from build123d import *

# Parameters (mm, degrees)
F0_W     = 38
F0_H     = 10
F1_DEPTH = 5
F2_R     = 1.5
F3_DEPTH = 5
F4_W     = 8
F4_H     = 5
F5_DEPTH = 5
F6_R     = 1.5
F7_DEPTH = 5
F8_R     = 4.99999


# Not quite as in the source:
# - a fillet or chamfer is up to 0.001 mm smaller than in the source, because OpenCascade refuses the exact size
# - a feature names something its author has since deleted; it is built from what else it names


with BuildPart() as f1:
    # F0 (on Top) → F1 (new body)
    with BuildSketch(Plane.XY):
        Polygon((20, -50), (20, 50), (-20, 50), (-20, 40), (-20, 12), (-20, 10), (-20, -50), align=None)
        with Locations((-39, 45)):
            Rectangle(F0_W, F0_H)
        Polygon((-58, 40), (-58, 50), (-60, 50), (-60, 10), (-20, 10), (-20, 12), (-58, 12), align=None)
    extrude(amount=F1_DEPTH)

    # F2 (on face) → F3 (cut)
    with BuildSketch(Plane.XY.offset(5)):
        with Locations((-35, 42)):
            Circle(F2_R)
        with Locations((-5, 15.5)):
            Circle(F2_R)
    extrude(amount=-F3_DEPTH, mode=Mode.SUBTRACT)

    # F4 (on face) → F5 (join)
    with BuildSketch(Plane.XY.offset(5)):
        with Locations((16, 47.5)):
            Rectangle(F4_W, F4_H)
        with Locations((-56, 47.5)):
            Rectangle(F4_W, F4_H)
    extrude(amount=F5_DEPTH)

    # F6 (on face) → F7 (cut)
    with BuildSketch(Plane(origin=(0, 50, 0), x_dir=(-1, 0, 0), z_dir=(0, 1, 0))):
        with BuildLine():
            ThreePointArc((-14.5, 7.5), (-14.9393398282, 8.5606601718), (-16, 9))
            ThreePointArc((-16, 9), (-17.0606601718, 6.4393398282), (-14.5, 7.5))
        make_face()
        with Locations((56, 7.5)):
            Circle(F6_R)
    extrude(amount=-F7_DEPTH, mode=Mode.SUBTRACT)

    # F8 (radius 5 in the source; OpenCascade refuses exactly that, so slightly less here)
    f8_edges = [f1.edges().sort_by_distance(p)[0] for p in [
        (-60, 10, 2.5),
        (-58, 12, 2.5),
        (-20, -20, 5),
        (-20, 26, 5),
        (0, -50, 5),
        (20, -2.5, 5),
        (-20, -50, 2.5),
        (20, -50, 2.5),
    ]]
    fillet(f8_edges, radius=F8_R)


solid = f1.part
Geometry: final body of the model. Coordinates: model frame, mm. A direction names the side the tool comes from. Round coordinates to 2 decimals unless told otherwise and drop trailing zeros. Loops run counter-clockwise (first coordinate to the right, second up) from the corner with the lowest first, then second, coordinate; pieces in that order, holes last. Notation, with made-up numbers: (-2, 40) -> (5, 40) arc R8 ccw to (5, 54) -> close; hole circle Ø10 at (-14, -21.75). An arc over 180 degrees is marked (long way). One line per question, with ' | ' between items. Start each with the question number.
1. Set-up query: faces 1 (the face through (-52, 47, 7)), 2 (the face through (-18, -18, 4)), 3 (the face through (-3, 12, 0)), 4 (the face through (-18, 26, 4)), 5 (the face through (-58, 28, 2)). Return all of +Z, -Z, +X, -X, +Y, -Y with unobstructed straight access to the full face (end or side cutting, diameter ignored); none if empty.
2. Section D-D on x = -35. Output: boundary loops of the cut face in (y, z).
3. Line query: line 1 along Y through (x, z) = (-35, 3.6); line 2 along Z through (x, y) = (16, 48.75); line 3 along Y through (x, z) = (-39, 0.5). Output: solid intervals per line, ascending. Write a range as [from, to].
4. Section C-C on z = 3.25. Output: boundary loops of the cut face in (x, y), and give its area (3 significant figures).
5. Contact query for flat-ended pins moving along their axis: pin 1 (4 mm diameter, centred on x = -31.5, z = 2.5, fed in from -Y); pin 2 (2.5 mm diameter, centred on y = 25, z = 3, fed in from +X); pin 3 (5 mm diameter, centred on x = -35, y = 42, fed in from +Z); pin 4 (3.5 mm diameter, centred on x = 16, z = 7.5, fed in from +Y). Output: stop coordinate, or through.
6. Section A-A on x = -43.5. Output: boundary loops of the cut face in (y, z), and give its area (3 significant figures).
7. Mould query, pull axis Y, two halves, no side actions, for faces 6 (the face through (17, 45, 6)), 7 (the face through (-57, 14, 3)), 8 (the face through (-57.386, 47.535, 6.925)). Classes: pulls with the +Y half, pulls with the -Y half, needs draft (parallel to the pull), parting line crosses it, or undercut.
Returned:
1) face 1: +Z, +Y, -Y | face 2: +Z, -X, -Y | face 3: -Z, +X, -X, +Y, -Y | face 4: +Z | face 5: +Z, -Z
2) outline: (10, 0) -> (12, 0) -> (12, 5) -> (10, 5) -> close; (40, 0) -> (40.5, 0) -> (40.5, 5) -> (40, 5) -> close; (43.5, 0) -> (50, 0) -> (50, 5) -> (43.5, 5) -> close
3) line 1: y = [10, 12], [40, 40.5], [43.5, 50] | line 2: z = [0, 6], [9, 10] | line 3: y = [10, 12], [40, 50]
4) outline: (-60, 15) arc R5 ccw to (-55, 10) -> (-18.8, 10) -> (-18.8, -45) arc R3.8 ccw to (-15, -48.8) -> (15, -48.8) arc R3.8 ccw to (18.8, -45) -> (18.8, 45) -> (20, 45) -> (20, 50) -> (-60, 50) -> close; hole (-58, 17) arc R5 ccw to (-53, 12) -> (-18.8, 12) -> (-18.8, 40) -> (-58, 40) -> close; hole circle Ø3 at (-35, 42); hole circle Ø3 at (-5, 15.5) | area: 4,250 mm2
5) pin 1: stops at y = 10 | pin 2: stops at x = 19.68 | pin 3: stops at z = 5 | pin 4: stops at y = 50
6) outline: (10, 0) -> (12, 0) -> (12, 5) -> (10, 5) -> close; (40, 0) -> (50, 0) -> (50, 5) -> (40, 5) -> close | area: 60.0 mm2
7) face 6: pulls with the -Y half | face 7: undercut | face 8: needs draft
